from build123d import *

# Parameters (mm, degrees)
SKETCH1_R                = 0.425
BOSS_EXTRUDE1_DEPTH      = 1.6
LPATTERN2_START          = -0.0125
LPATTERN2_OUTLINE_R      = 0.425
LPATTERN2_DEPTH          = 1.6
SLOTFOOTPRINTS_REF_DEPTH = 0.0001
SLOTFOOTPRINTS_DEPTH     = 0.0001
SKETCH2_R                = 0.8
F_20PIN_MOUNTS_DEPTH     = 71.235674696
SKETCH3_R                = 0.8
F_12PIN_MOUNTS_DEPTH     = 10
SKETCH4_R                = 25
CUT_EXTRUDE1_DEPTH       = 71.235674696


# Read off the part's stored shape, not the designer's step: LPattern2
with BuildPart() as part:
    # Sketch1 → Boss-Extrude1 (new body)
    with BuildSketch(Plane(origin=(0, 0, -0.0125), x_dir=(-1, 0, 0), z_dir=(0, 0, -1))):
        with BuildLine():
            Line((35.3, -50), (35.3, -48))
            ThreePointArc((35.3, -48), (35.592893219, -47.292893219), (36.3, -47))
            Line((36.3, -47), (45.8, -47))
            ThreePointArc((45.8, -47), (46.507106781, -46.707106781), (46.8, -46))
            Line((46.8, -46), (46.8, -41.4))
            ThreePointArc((46.8, -41.4), (47.092893219, -40.692893219), (47.8, -40.4))
            Line((47.8, -40.4), (49.3, -40.4))
            Line((49.3, -40.4), (49.3, 39.2))
            Line((49.3, 39.2), (43.2, 45.3))
            Line((43.2, 45.3), (35.500000002, 45.3))
            Line((35.500000002, 45.3), (3.499999998, 45.3))
            Line((3.499999998, 45.3), (-43.2, 45.3))
            Line((-43.2, 45.3), (-49.3, 39.2))
            Line((-49.3, 39.2), (-49.3, -40.4))
            Line((-49.3, -40.4), (-47.8, -40.4))
            ThreePointArc((-47.8, -40.4), (-47.092893219, -40.692893219), (-46.8, -41.4))
            Line((-46.8, -41.4), (-46.8, -46))
            ThreePointArc((-46.8, -46), (-46.507106781, -46.707106781), (-45.8, -47))
            Line((-45.8, -47), (-36.3, -47))
            ThreePointArc((-36.3, -47), (-35.592893219, -47.292893219), (-35.3, -48))
            Line((-35.3, -48), (-35.3, -50))
            Line((-35.3, -50), (35.3, -50))
        make_face()
        with Locations(Location((-21.27, 41.37, 0), (0, 0, 180))):
            Circle(SKETCH1_R, mode=Mode.SUBTRACT)
        with Locations(Location((-23.81, 41.37, 0), (0, 0, 180))):
            Circle(SKETCH1_R, mode=Mode.SUBTRACT)
        with Locations(Location((-22.54, 40.1, 0), (0, 0, 180))):
            Circle(SKETCH1_R, mode=Mode.SUBTRACT)
        with Locations(Location((-13.87, 41.37, 0), (0, 0, 180))):
            Circle(SKETCH1_R, mode=Mode.SUBTRACT)
        with Locations(Location((-23.81, 38.83, 0), (0, 0, 180))):
            Circle(SKETCH1_R, mode=Mode.SUBTRACT)
        with Locations(Location((-16.41, 41.37, 0), (0, 0, 180))):
            Circle(SKETCH1_R, mode=Mode.SUBTRACT)
        with Locations(Location((-15.14, 40.1, 0), (0, 0, 180))):
            Circle(SKETCH1_R, mode=Mode.SUBTRACT)
        with Locations(Location((-21.27, 38.83, 0), (0, 0, 180))):
            Circle(SKETCH1_R, mode=Mode.SUBTRACT)
        with Locations(Location((-28.67, 41.37, 0), (0, 0, 180))):
            Circle(SKETCH1_R, mode=Mode.SUBTRACT)
        with Locations(Location((-31.21, 41.37, 0), (0, 0, 180))):
            Circle(SKETCH1_R, mode=Mode.SUBTRACT)
        with Locations(Location((-16.41, 38.83, 0), (0, 0, 180))):
            Circle(SKETCH1_R, mode=Mode.SUBTRACT)
        with Locations(Location((-29.94, 40.1, 0), (0, 0, 180))):
            Circle(SKETCH1_R, mode=Mode.SUBTRACT)
        with Locations(Location((-31.21, 38.83, 0), (0, 0, 180))):
            Circle(SKETCH1_R, mode=Mode.SUBTRACT)
        with Locations(Location((-28.67, 38.83, 0), (0, 0, 180))):
            Circle(SKETCH1_R, mode=Mode.SUBTRACT)
        with Locations(Location((-13.87, 38.83, 0), (0, 0, 180))):
            Circle(SKETCH1_R, mode=Mode.SUBTRACT)
    extrude(amount=-BOSS_EXTRUDE1_DEPTH)

    # LPattern2 outline → LPattern2 (cut)
    with BuildSketch(Plane.XY.offset(LPATTERN2_START)):
        with Locations((31.21, 31.37)):
            Circle(LPATTERN2_OUTLINE_R)
        with Locations((31.21, 28.83)):
            Circle(LPATTERN2_OUTLINE_R)
        with Locations((29.94, 30.1)):
            Circle(LPATTERN2_OUTLINE_R)
        with Locations((28.67, 28.83)):
            Circle(LPATTERN2_OUTLINE_R)
        with Locations((28.67, 31.37)):
            Circle(LPATTERN2_OUTLINE_R)
        with Locations((16.41, 31.37)):
            Circle(LPATTERN2_OUTLINE_R)
        with Locations((23.81, 31.37)):
            Circle(LPATTERN2_OUTLINE_R)
        with Locations((23.81, 28.83)):
            Circle(LPATTERN2_OUTLINE_R)
        with Locations((22.54, 30.1)):
            Circle(LPATTERN2_OUTLINE_R)
        with Locations((21.27, 28.83)):
            Circle(LPATTERN2_OUTLINE_R)
        with Locations((21.27, 31.37)):
            Circle(LPATTERN2_OUTLINE_R)
        with Locations((16.41, 28.83)):
            Circle(LPATTERN2_OUTLINE_R)
        with Locations((15.14, 30.1)):
            Circle(LPATTERN2_OUTLINE_R)
        with Locations((13.87, 28.83)):
            Circle(LPATTERN2_OUTLINE_R)
        with Locations((13.87, 31.37)):
            Circle(LPATTERN2_OUTLINE_R)
    extrude(amount=LPATTERN2_DEPTH, mode=Mode.SUBTRACT)

    # thermalContacts_lower → slotFootprints_REF (cut)
    with BuildSketch(Plane(origin=(0, 0, -0.0125), x_dir=(-1, 0, 0), z_dir=(0, 0, -1))):
        Polygon((47, 35.5), (47, -41.5), (59.827263463, -41.5), (59.827263463, 47), (41.5, 47), (41.5, 41.5), (41.5, 35.5), align=None)
        Polygon((-47, 35.5), (-47, -41.5), (-56.192158269, -41.5), (-56.192158269, 47), (-41.5, 47), (-41.5, 41.5), (-41.5, 35.5), align=None)
    extrude(amount=-SLOTFOOTPRINTS_REF_DEPTH, mode=Mode.SUBTRACT)

    # thermalContacts_upper → slotFootprints (cut)
    with BuildSketch(Plane.XY.offset(1.5875)):
        Polygon((-47, 35.5), (-47, -41.5), (-56.192158269, -41.5), (-56.192158269, 47), (-41.5, 47), (-41.5, 41.5), (-41.5, 35.5), align=None)
        Polygon((47, 35.5), (47, -41.5), (59.827263463, -41.5), (59.827263463, 47), (41.5, 47), (41.5, 41.5), (41.5, 35.5), align=None)
    extrude(amount=-SLOTFOOTPRINTS_DEPTH, mode=Mode.SUBTRACT)

    # Sketch2 → 20pin_mounts (cut, through all)
    with BuildSketch(Plane.XY.offset(1.5875)):
        with Locations((-33.775, 38.472296419)):
            Circle(SKETCH2_R)
        with Locations((-17.925, 38.472296419)):
            Circle(SKETCH2_R)
        with Locations((-17.925, 28.472296419)):
            Circle(SKETCH2_R)
        with Locations((-33.775, 28.472296419)):
            Circle(SKETCH2_R)
        with BuildLine():
            Line((-35.775, 45.3), (-35.775, 43.8))
            ThreePointArc((-35.775, 43.8), (-35.482106781, 43.092893219), (-34.775, 42.8))
            Line((-34.775, 42.8), (-16.925, 42.8))
            ThreePointArc((-16.925, 42.8), (-16.217893218, 43.092893219), (-15.925, 43.8))
            Line((-15.925, 43.8), (-15.925, 45.3))
            Line((-15.925, 45.3), (-35.775, 45.3))
        make_face()
    extrude(amount=-F_20PIN_MOUNTS_DEPTH, mode=Mode.SUBTRACT)

    # Sketch3 → 12pin_mounts (cut)
    with BuildSketch(Plane(origin=(0, 0, -0.0125), x_dir=(-1, 0, 0), z_dir=(0, 0, -1))):
        with Locations((5.390000006, 41.4)):
            Circle(SKETCH3_R)
        with Locations((-5.379999994, 41.4)):
            Circle(SKETCH3_R)
        with Locations((43.1, 5.379999994)):
            Circle(SKETCH3_R)
        with Locations((43.1, -5.390000006)):
            Circle(SKETCH3_R)
        with Locations((5.390000006, -42.303202712)):
            Circle(SKETCH3_R)
        with Locations((-5.379999994, -42.303202712)):
            Circle(SKETCH3_R)
        with Locations((-43.1, -5.390000006)):
            Circle(SKETCH3_R)
        with Locations((-43.1, 5.379999994)):
            Circle(SKETCH3_R)
        with BuildLine():
            Line((-49.3, 7.379999994), (-48, 7.379999994))
            ThreePointArc((-48, 7.379999994), (-47.292893219, 7.087106775), (-47, 6.379999994))
            Line((-47, 6.379999994), (-47, -6.390000006))
            ThreePointArc((-47, -6.390000006), (-47.292893219, -7.097106787), (-48, -7.390000006))
            Line((-48, -7.390000006), (-49.3, -7.390000006))
            Line((-49.3, -7.390000006), (-49.3, 7.379999994))
        make_face()
        with BuildLine():
            Line((48, 7.379999994), (49.3, 7.379999994))
            Line((49.3, 7.379999994), (49.3, -7.390000006))
            Line((49.3, -7.390000006), (48, -7.390000006))
            ThreePointArc((48, -7.390000006), (47.292893219, -7.097106787), (47, -6.390000006))
            Line((47, -6.390000006), (47, 6.379999994))
            ThreePointArc((47, 6.379999994), (47.292893219, 7.087106775), (48, 7.379999994))
        make_face()
        with BuildLine():
            Line((-6.379999994, -46.203202712), (6.390000006, -46.203202712))
            ThreePointArc((6.390000006, -46.203202712), (7.097106787, -46.496095931), (7.390000006, -47.203202712))
            Line((7.390000006, -47.203202712), (7.390000006, -50))
            Line((7.390000006, -50), (-7.379999994, -50))
            Line((-7.379999994, -50), (-7.379999994, -47.203202712))
            ThreePointArc((-7.379999994, -47.203202712), (-7.087106775, -46.496095931), (-6.379999994, -46.203202712))
        make_face()
    extrude(amount=-F_12PIN_MOUNTS_DEPTH, mode=Mode.SUBTRACT)

    # Sketch4 → Cut-Extrude1 (cut, through all)
    with BuildSketch(Plane(origin=(0, 0, -0.0125), x_dir=(-1, 0, 0), z_dir=(0, 0, -1))):
        Circle(SKETCH4_R)
    extrude(amount=-CUT_EXTRUDE1_DEPTH, mode=Mode.SUBTRACT)


solid = part.part
Read the model definition and answer for the solid it produces. Units are mm, in the model's axes. Give positions to 0.01 mm unless a question says otherwise; leave off trailing zeros. Write each loop counter-clockwise with the first axis right and the second up, starting at its lowest first coordinate (ties: lowest second). Pieces come first, ordered by that corner, then holes. Notation, with made-up numbers: M -32,81.5 L -25,81.5 A17 ccw -25,97.5 Z; hole C -12,27.25 d1. An arc over 180 degrees is marked long. One line per item, written item: value. Start each with the question number.
(1) Flat-ended cylindrical pins translate along their axes: pin 1 Ø0.8 at (y, z) = (-49, 1) entering from -X; pin 2 Ø0.5 at (y, z) = (-43.5, 1) entering from -X; pin 3 Ø1.4 at (x, y) = (-43.1, 5.38) entering from +Z; pin 4 Ø0.6 at (x, z) = (-48.5, 1) entering from -Y. Find the tip coordinate at first contact, or state that the pin passes through.
(2) Find section A-A (y = 0). Determine the outline of the cut face in (x, z), plus the area to 3 significant figures.
(3) Find section B-B (x = -21.5). Determine the outline of the cut face in (y, z), plus the area to 3 significant figures.
(4) Find section D-D (z = 1.15). Give the number of separate pieces and of enclosed holes in the cut face, plus the area to 3 significant figures.
(5) Find the intervals of material crossed by line 1 (Y direction, x = 43.1, z = 0.5); line 2 (Y direction, x = 31.21, z = 0.9) (3 decimals); line 3 (X direction, y = 6, z = 1), in increasing order.
(6) Determine the mould class of faces 1 (the flat face through (48, -23, -0.012)), 2 (the cylindrical face through (-23.846, 7.509, 0.776)), 3 (the flat face through (-46.3, 42.2, 0.8)) for opening direction Y: pulls with the +Y half, pulls with the -Y half, needs draft (parallel to the pull), parting line crosses it, or undercut.
Results below:
1. pin 1: stops at x = -35.3
1. pin 2: stops at x = -46.8
1. pin 3: passes through
1. pin 4: stops at y = -40.4
2. outline: M -47,-0.01 L -25,-0.01 L -25,1.59 L -47,1.59 Z; M 25,-0.01 L 47,-0.01 L 47,1.59 L 25,1.59 Z
2. area: 70.4 mm^2
3. outline: M -50,-0.01 L -12.76,-0.01 L -12.76,1.59 L -50,1.59 Z; M 12.76,-0.01 L 42.8,-0.01 L 42.8,1.59 L 12.76,1.59 Z
3. area: 108 mm^2
4. separate pieces: 1
4. enclosed holes: 43
4. area: 7,070 mm^2
5. line 1: y = -47 to -6.19, -4.59 to 4.58, 6.18 to 45.3
5. line 2: y = -50 to 28.405, 29.255 to 30.945, 31.795 to 38.405, 39.255 to 40.945, 41.795 to 45.3
5. line 3: x = -47 to -43.61, -42.59 to -24.27, 24.27 to 42.59, 43.61 to 47
6. face 1: needs draft
6. face 2: undercut
6. face 3: pulls with the +Y half
